from build123d import *

# Parameters (mm, degrees)
SKETCH_W     = 70
SKETCH_H     = 80
PAD_DEPTH    = 2
PAD001_DEPTH = 12.5
PAD002_DEPTH = 4
FILLET_R     = 10


with BuildPart() as part:
    # Sketch → Pad (new body, symmetric)
    with BuildSketch(Plane.XZ):
        Rectangle(SKETCH_W, SKETCH_H)
    extrude(amount=PAD_DEPTH, both=True)

    # Sketch001 → Pad001 (join, symmetric)
    with BuildSketch(Plane.YZ):
        Polygon((0, 25), (-35, 25), (-76.954982, -25), (-71.733352, -25), (-32.690599, 21), (0, 21), align=None)
    extrude(amount=PAD001_DEPTH, both=True)

    # Sketch002 (on Face7 of Pad001) → Pad002 (join)
    with BuildSketch(Plane(origin=(12.5, 0, 0), x_dir=(0, 0, 1), z_dir=(1, 0, 0))):
        Polygon((-25, 76.954982), (-25, 0), (25, 0), (25, 35), align=None)
    pad002 = extrude(amount=PAD002_DEPTH)

    # Mirrored: Pad002 across YZ
    add(pad002.mirror(Plane.YZ))

    # Fillet
    fillet_edges = [part.edges().sort_by_distance(p)[0] for p in [
        (35, 0, 40),
        (35, 0, -40),
        (-35, 0, 40),
        (-35, 0, -40),
    ]]
    fillet(fillet_edges, radius=FILLET_R)


solid = part.part
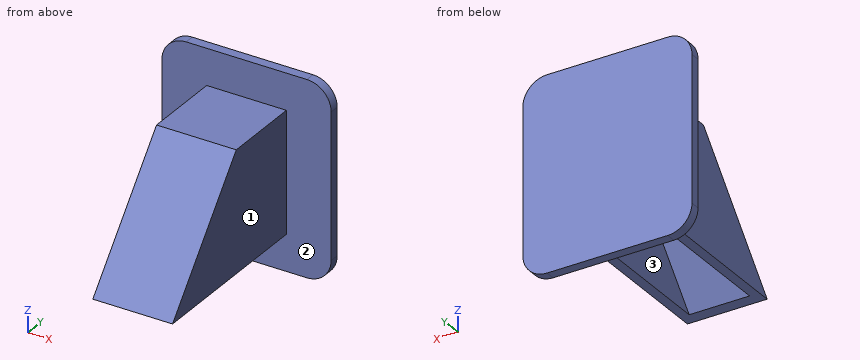
For this review, take the finished solid that the model builds, in its own axes (mm). Face numbers are marked on the shaded views. A direction names the side the tool comes from. Round coordinates to 2 decimals unless told otherwise and drop trailing zeros. Order: outer loops, then holes, each group sorted by start corner. A loop starts at its lowest first (then second) coordinate and runs counter-clockwise, first axis right, second up. Notation, with made-up numbers: (7, 61.5) -> (48, 61.5) arc R21 ccw to (48, 99.5) -> close; hole circle Ø8 at (-31, 44). An arc over 180 degrees is marked (long way). Write item = value, one per line. Start each with the question number.
1) Take a section at C-C on x = 22. State the section outline as (y, z) points.
2) Take a section at A-A on y = -6.5. State the section outline as (x, z) points.
3) Take a section at B-B on z = 19. State the section outline as (x, y) points.
4) Insertion check: pin 1 (5 mm diameter, centred on y = -31.5, z = 24, fed in from +X); pin 2 (8 mm diameter, centred on x = 5, z = 7, fed in from -Y); pin 3 (20 mm diameter, centred on x = 4, y = -12.5, fed in from -Z). Each pin has a flat end and moves straight along its axis. Give the tip position at first contact, or say it passes through.
5) To check wall thickness, follow line 1 (X direction, y = -16, z = 8); line 2 (Y direction, x = 17.5, z = 30); line 3 (Z direction, x = -13, y = -11.5). State the ranges of each line that lie inside material, in increasing order. Write a range as from..to.
6) Tool access review of the marked faces 1, 2 and 3: name each direction out of +Z, -Z, +X, -X, +Y, -Y from which nothing blocks a thin tool from reaching the whole face with its end or side.
7) Take a section at D-D on z = -1.5. State the section outline as (x, y) points.
Verdict:
q1.outline = (-2, -40) -> (2, -40) -> (2, 40) -> (-2, 40) -> close
q2.outline = (-16.5, -25) -> (-12.5, -25) -> (-12.5, 21) -> (12.5, 21) -> (12.5, -25) -> (16.5, -25) -> (16.5, 25) -> (-16.5, 25) -> close
q3.outline = (-35, -2) -> (-16.5, -2) -> (-16.5, -40.03) -> (16.5, -40.03) -> (16.5, -2) -> (35, -2) -> (35, 2) -> (-35, 2) -> close; hole (-12.5, -34.39) -> (12.5, -34.39) -> (12.5, -2) -> (-12.5, -2) -> close
q4.pin_1 = 16.5
q4.pin_2 = -53.46
q4.pin_3 = -25
q5.line_1 = -16.5..-12.5, 12.5..16.5
q5.line_2 = -2..2
q5.line_3 = -25..25
q6.face_1 = +Z, -Z, +X, -Y
q6.face_2 = none
q6.face_3 = -Z
q7.outline = (-35, -2) -> (-16.5, -2) -> (-16.5, -57.24) -> (16.5, -57.24) -> (16.5, -2) -> (35, -2) -> (35, 2) -> (-35, 2) -> close; hole (-12.5, -51.79) -> (12.5, -51.79) -> (12.5, -2) -> (-12.5, -2) -> close
